Part model, mm, in its own coordinate system. Round coordinates to 2 decimals unless told otherwise and drop trailing zeros. Write each loop counter-clockwise with the first axis right and the second up, starting at its lowest first coordinate (ties: lowest second). Pieces come first, ordered by that corner, then holes. Notation, with made-up numbers: (21.5, -27) -> (46.5, -27) arc R22 cw to (46.5, 9) -> close; hole circle Ø6 at (82.5, 36.5). An arc over 180 degrees is marked (long way). Use CSV: the item, a comma, the result in double quotes. Start each with the question number.
(1) Drop flat-ended pins along their axis: pin 1 (2.5 mm diameter, centred on x = 37.52, y = -52.5, fed in from -Z); pin 2 (0.9 mm diameter, centred on y = -81, z = 2, fed in from +X). Give the stop position or say it passes through.
(2) Saw through at C-C (x = 60.9). Give the cut face in (y, z), plus the area to 3 significant figures.
(3) Probe line 1 (Y direction, x = 116.5, z = 1.4); line 2 (X direction, y = -38.5, z = 2.2); line 3 (Y direction, x = 60.9, z = 2.3). List the from-to ranges inside material, lowest first. Write a range as [from, to].
(4) Saw through at D-D (x = 115). Give the cut face in (y, z), plus the area to 3 significant figures.
(5) Saw through at B-B (z = 2.15). Count the separate pieces of the cut face and the enclosed holes in it, plus the area to 3 significant figures.
(6) Saw through at A-A (y = -37.5). Give the cut face in (x, z), plus the area to 3 significant figures.
```python
from build123d import *

# Parameters (mm, degrees)
EXTRUDE_1_DEPTH     = 3
CUT_EXTRUDE_1_REACH = 236.261
SKETCH_2_R          = 2.15
CHAMFER_1_SIZE      = 13
CHAMFER_1_SIZE2     = 8
CHAMFER_2_SIZE      = 8
CHAMFER_2_SIZE2     = 13
SKETCH_6_R          = 5
CUT_EXTRUDE_4_DEPTH = 10
SKETCH_7_R          = 2.15
CUT_EXTRUDE_5_DEPTH = 235.260538717


with BuildPart() as part:
    # 草图1 → 凸台-拉伸1 (new body)
    with BuildSketch(Plane.XY):
        with BuildLine():
            Line((0, 0), (0, -60))
            Line((0, -60), (53, -60))
            Line((53, -60), (53, -110))
            ThreePointArc((53, -110), (60.908116908, -129.091883092), (80, -137))
            Line((80, -137), (110, -137))
            ThreePointArc((110, -137), (129.091883092, -129.091883092), (137, -110))
            Line((137, -110), (137, -60))
            Line((137, -60), (190, -60))
            Line((190, -60), (190, 0))
            Line((190, 0), (0, 0))
        make_face()
    extrude(amount=EXTRUDE_1_DEPTH)

    # 草图2 → 切除-拉伸1 (cut, up to next)
    with BuildSketch(Plane.XY.offset(3), mode=Mode.PRIVATE) as cut_extrude_1_sk1:
        with Locations((75, -115)):
            Circle(SKETCH_2_R)
    cut_extrude_1_tool1 = extrude(cut_extrude_1_sk1.sketch, amount=-CUT_EXTRUDE_1_REACH, mode=Mode.PRIVATE) & part.part
    # 草图2 → 切除-拉伸1 (cut, up to next)
    with BuildSketch(Plane.XY.offset(3), mode=Mode.PRIVATE) as cut_extrude_1_sk2:
        with Locations((115, -115)):
            Circle(SKETCH_2_R)
    cut_extrude_1_tool2 = extrude(cut_extrude_1_sk2.sketch, amount=-CUT_EXTRUDE_1_REACH, mode=Mode.PRIVATE) & part.part
    add(cut_extrude_1_tool1.solids().sort_by_distance((75, -115, 3))[0], mode=Mode.SUBTRACT)
    add(cut_extrude_1_tool2.solids().sort_by_distance((115, -115, 3))[0], mode=Mode.SUBTRACT)

    # 倒角1
    chamfer_1_edges = [part.edges().sort_by_distance(p)[0] for p in [
        (53, -60, 1.5),
    ]]
    chamfer_1_side = [part.faces().sort_by_distance(p)[0] for p in [
        (26.5, -60, 1.5),
    ]]
    chamfer(chamfer_1_edges, length=CHAMFER_1_SIZE, length2=CHAMFER_1_SIZE2, reference=chamfer_1_side[0])

    # 倒角2
    chamfer_2_edges = [part.edges().sort_by_distance(p)[0] for p in [
        (137, -60, 1.5),
    ]]
    chamfer_2_side = [part.faces().sort_by_distance(p)[0] for p in [
        (137, -85, 1.5),
    ]]
    chamfer(chamfer_2_edges, length=CHAMFER_2_SIZE, length2=CHAMFER_2_SIZE2, reference=chamfer_2_side[0])

    # 草图6 → 切除-拉伸4 (cut)
    with BuildSketch(Plane(origin=(0, 0, 0), x_dir=(-1, 0, 0), z_dir=(0, 0, -1))):
        with Locations((-117.79084048, -81)):
            Circle(SKETCH_6_R)
    extrude(amount=-CUT_EXTRUDE_4_DEPTH, mode=Mode.SUBTRACT)

    # 草图7 → 切除-拉伸5 (cut, through all)
    with BuildSketch(Plane(origin=(0, 0, 0), x_dir=(-1, 0, 0), z_dir=(0, 0, -1))):
        with Locations((-129.1, -7.5)):
            Circle(SKETCH_7_R)
        with Locations((-152.48, -7.5)):
            Circle(SKETCH_7_R)
        with Locations((-152.48, -22.5)):
            Circle(SKETCH_7_R)
        with Locations((-129.1, -22.5)):
            Circle(SKETCH_7_R)
        with Locations((-152.48, -37.5)):
            Circle(SKETCH_7_R)
        with Locations((-129.1, -37.5)):
            Circle(SKETCH_7_R)
        with Locations((-152.48, -52.5)):
            Circle(SKETCH_7_R)
        with Locations((-129.1, -52.5)):
            Circle(SKETCH_7_R)
        with Locations((-60.9, -22.5)):
            Circle(SKETCH_7_R)
        with Locations((-37.52, -22.5)):
            Circle(SKETCH_7_R)
        with Locations((-60.9, -37.5)):
            Circle(SKETCH_7_R)
        with Locations((-37.52, -37.5)):
            Circle(SKETCH_7_R)
        with Locations((-60.9, -52.5)):
            Circle(SKETCH_7_R)
        with Locations((-37.52, -52.5)):
            Circle(SKETCH_7_R)
        with Locations((-60.9, -7.5)):
            Circle(SKETCH_7_R)
        with Locations((-37.52, -7.5)):
            Circle(SKETCH_7_R)
    extrude(amount=-CUT_EXTRUDE_5_DEPTH, mode=Mode.SUBTRACT)


solid = part.part
```
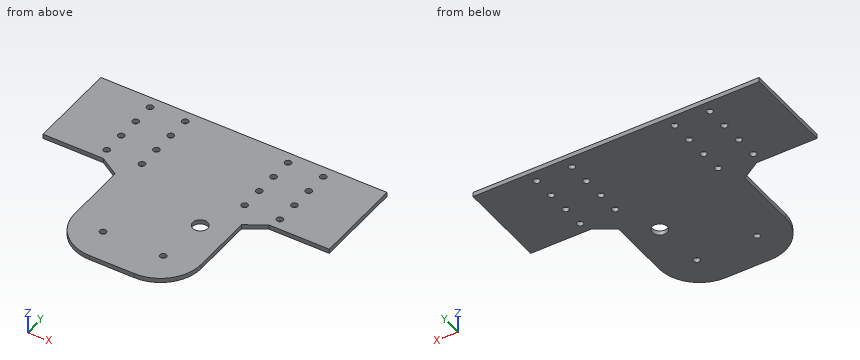
Answers:
1,pin 1,"passes through"
1,pin 2,"stops at x = 137"
2,outline,"(-129.08, 0) -> (-54.65, 0) -> (-54.65, 3) -> (-129.08, 3) -> close; (-50.35, 0) -> (-39.65, 0) -> (-39.65, 3) -> (-50.35, 3) -> close; (-35.35, 0) -> (-24.65, 0) -> (-24.65, 3) -> (-35.35, 3) -> close; (-20.35, 0) -> (-9.65, 0) -> (-9.65, 3) -> (-20.35, 3) -> close; (-5.35, 0) -> (0, 0) -> (0, 3) -> (-5.35, 3) -> close"
2,area,"336 mm²"
3,line 1,"y = [-136.21, -116.54], [-113.46, -85.83], [-76.17, 0]"
3,line 2,"x = [0, 35.62], [39.42, 59], [62.8, 127.2], [131, 150.58], [154.38, 190]"
3,line 3,"y = [-129.08, -54.65], [-50.35, -39.65], [-35.35, -24.65], [-20.35, -9.65], [-5.35, 0]"
4,outline,"(-136.53, 0) -> (-117.15, 0) -> (-117.15, 3) -> (-136.53, 3) -> close; (-112.85, 0) -> (-85.15, 0) -> (-85.15, 3) -> (-112.85, 3) -> close; (-76.85, 0) -> (0, 0) -> (0, 3) -> (-76.85, 3) -> close"
4,area,"372 mm²"
5,separate pieces,"1"
5,enclosed holes,"19"
5,area,"17,300 mm²"
6,outline,"(0, 0) -> (35.37, 0) -> (35.37, 3) -> (0, 3) -> close; (39.67, 0) -> (58.75, 0) -> (58.75, 3) -> (39.67, 3) -> close; (63.05, 0) -> (126.95, 0) -> (126.95, 3) -> (63.05, 3) -> close; (131.25, 0) -> (150.33, 0) -> (150.33, 3) -> (131.25, 3) -> close; (154.63, 0) -> (190, 0) -> (190, 3) -> (154.63, 3) -> close"
6,area,"518 mm²"
